For this review, take the finished solid that the model builds, in its own axes (mm). Face numbers are marked on the shaded views. A direction names the side the tool comes from. Coordinates: 2 decimals unless noted, no trailing zeros. Loops run counter-clockwise (first coordinate to the right, second up) from the corner with the lowest first, then second, coordinate; pieces in that order, holes last.
```python
from build123d import *

# Parameters (mm, degrees)
CHAMFER1_SIZE      = 0.625
CUT_EXTRUDE1_DEPTH = 4
CHAMFER2_SIZE      = 0.8
FILLET1_R          = 0.4


with BuildPart() as part:
    # Sketch1 → Revolve1 (revolve)
    with BuildSketch(Plane(origin=(0, 0, 0), x_dir=(1, 0, 0), z_dir=(0, 1, 0))):
        Polygon((0, 0), (0, 4), (5, 4), (5, 2), (25, 2), (25, 0), align=None)
    revolve(axis=Axis((25, 0, 0), (-1, 0, 0)))

    # Chamfer1
    chamfer1_edges = [part.edges().sort_by_distance(p)[0] for p in [
        (25, 0, 2),
    ]]
    chamfer(chamfer1_edges, length=CHAMFER1_SIZE)

    # Sketch3 → Cut-Revolve1 (revolve, cut)
    with BuildSketch(Plane(origin=(0, 0, 0), x_dir=(1, 0, 0), z_dir=(0, 1, 0)), mode=Mode.PRIVATE) as cut_revolve1_sk:
        Polygon((0, 0), (5.732050808, 0), (4, 3), (0, 3), align=None)
    revolve(cut_revolve1_sk.sketch.rotate(Axis((0, 0, 0), (1, 0, 0)), 180), axis=Axis((0, 0, 0), (1, 0, 0)), mode=Mode.SUBTRACT)

    # Sketch2 → Cut-Extrude1 (cut)
    with BuildSketch(Plane.ZY):
        Polygon((0, 3.464101615), (-3, 1.732050808), (-3, -1.732050808), (0, -3.464101615), (3, -1.732050808), (3, 1.732050808), align=None)
    extrude(amount=-CUT_EXTRUDE1_DEPTH, mode=Mode.SUBTRACT)

    # Chamfer2
    # the kernel refuses this chamfer: 0.8 mm, written as the material it takes off along each edge
    with BuildSketch(Plane(origin=(0, 0, 0), x_dir=(0, 0, -1), z_dir=(0, 1, 0))) as chamfer2_piece_1:
        Polygon((4, -CHAMFER2_SIZE), (4 - CHAMFER2_SIZE, 0), (4, 0), align=None)
    revolve(axis=Axis((0, 0, 0), (-1, 0, 0)), mode=Mode.SUBTRACT)

    # Fillet1
    fillet1_edges = [part.edges().sort_by_distance(p)[0] for p in [
        (5, 0, 2),
    ]]
    fillet(fillet1_edges, radius=FILLET1_R)


solid = part.part
```
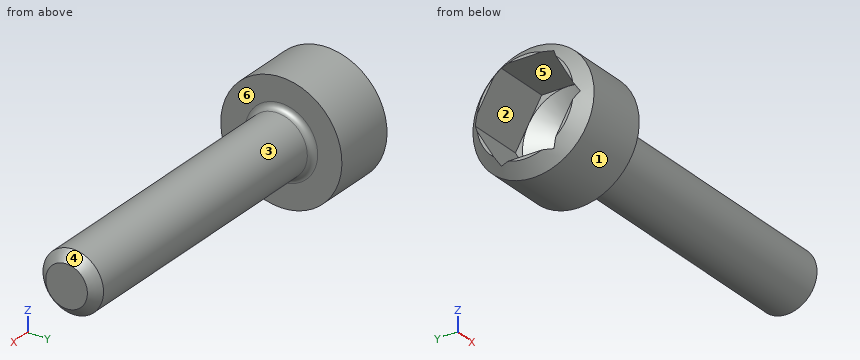
Q1. Wall thickness on probe 1 along Z at (x, y) = (7, 0); probe 2 along X at (y, z) = (3, -0.75); probe 3 along Y at (x, z) = (3.25, -1.75): over which ranges is each line inside the solid? List them lowest first.
Q2. The part is to be moulded in two halves that separate along Y. For the marked faces 4, 5 and 6, say which applies: +Y half, -Y half, draft (parallel to the pull), parting line (faces both ways), or undercut.
Q3. Consider section A-A (x = 11.75). State the section outline as (y, z) points, then the cut area to 3 significant figures.
Q4. For pin 1 Ø0.7 at (y, z) = (-3, 0.5) entering from -X; pin 2 Ø0.7 at (y, z) = (3, 0) entering from -X; pin 3 Ø3 at (x, z) = (9, 1.5) entering from -Y; pin 4 Ø2 at (x, z) = (14.5, 1.5) entering from +Y, all flat-tipped, find the tip position at first contact; note any pin that passes through.
Q5. Machinability: for the marked faces 1, 2 and 3, which of the approach directions +Z, -Z, +X, -X, +Y, -Y give a long, thin tool a straight path to every point of the face, cutting with its end or side? Answer none if there is none.
Model answer:
1. probe 1: z = -2 to 2
1. probe 2: x = 4 to 5
1. probe 3: y = -3.6 to -2.45, 2.45 to 3.6
2. face 4: parting line
2. face 5: undercut
2. face 6: draft
3. outline: circle Ø4 at (0, 0)
3. area: 12.6 mm2
4. pin 1: stops at x = 0
4. pin 2: stops at x = 4
4. pin 3: stops at y = -2
4. pin 4: stops at y = 1.94
5. face 1: +X, -X
5. face 2: -X
5. face 3: +X
